```python
from build123d import *

# Parameters (mm, degrees)
PAD002_DEPTH           = 4
SKETCH020_W            = 5
SKETCH020_H            = 30
POCKET003_DEPTH        = 4.001
POCKET003_DEPTH_BACK   = 4.001
FUSION_PLACEMENT_ANGLE = 35


with BuildPart() as obj1:
    # AdditivePipe003: sweep along a path in Sketch015
    with BuildLine(Plane.XZ) as additivepipe003_path:
        Line((0, -9), (10, -9))
        ThreePointArc((10, -9), (19, 2e-06), (9.999996, 9))
        Line((9.999996, 9), (0, 9))
    # Sketch016 → AdditivePipe003 (sweep)
    with BuildSketch(Plane.YZ):
        with BuildLine():
            ThreePointArc((-4, 9), (0, 5), (4, 9))
            Line((4, 11.082268), (4, 9))
            Line((1.261195, 13), (4, 11.082268))
            Line((-1.261195, 13), (1.261195, 13))
            Line((-1.261195, 13), (-4, 11.082268))
            Line((-4, 9), (-4, 11.082268))
        make_face()
    sweep(path=additivepipe003_path.line)

    # AdditivePipe004: sweep along a path in Sketch017
    with BuildLine(Plane.XZ) as additivepipe004_path:
        ThreePointArc((9, 9), (0, 0), (9, -9))
    # Sketch018 → AdditivePipe004 (sweep)
    with BuildSketch(Plane.YZ.offset(9)):
        with BuildLine():
            ThreePointArc((-4, 9), (0, 5), (4, 9))
            Line((4, 11.082268), (4, 9))
            Line((1.261195, 13), (4, 11.082268))
            Line((-1.261195, 13), (1.261195, 13))
            Line((-1.261195, 13), (-4, 11.082268))
            Line((-4, 9), (-4, 11.082268))
        make_face()
    sweep(path=additivepipe004_path.line)

    # Sketch019 → Pad002 (new body, symmetric)
    with BuildSketch(Plane.XZ):
        with BuildLine():
            Line((0, 10), (3.5, 10))
            Line((3.5, 10), (3.5, 8.351647))
            ThreePointArc((3.5, 8.351647), (-1, 0), (3.5, -8.351647))
            Line((3.5, -8.351647), (3.5, -10))
            Line((3.5, -10), (0, -10))
            Line((0, -10), (-2, 0))
            Line((0, 10), (-2, 0))
        make_face()
    extrude(amount=PAD002_DEPTH, both=True)

    # Sketch020 → Pocket003 (cut, two sides)
    with BuildSketch(Plane.XZ) as pocket003_sk:
        with Locations((-2.5, 0)):
            Rectangle(SKETCH020_W, SKETCH020_H)
    extrude(amount=-POCKET003_DEPTH, mode=Mode.SUBTRACT)
    extrude(pocket003_sk.sketch, amount=POCKET003_DEPTH_BACK, mode=Mode.SUBTRACT)


with BuildPart() as fat_link:
    # Part__Mirroring: instance of obj1
    add(obj1.part.mirror(Plane(origin=(0, 0, 0), x_dir=(0, -1, 0), z_dir=(1, 0, 0))))

    # Fusion: union obj1
    add(obj1.part)


with BuildPart() as fat_link_1:
    # Fusion placement: moved
    add(fat_link.part.rotate(Axis((0, 0, 0), (-1, 0, 0)), FUSION_PLACEMENT_ANGLE))


solid = fat_link_1.part
```
Verification items for the finished model (mm, model axes). A direction names the side the tool comes from. Give positions to 0.01 mm unless a question says otherwise; leave off trailing zeros. Use a Markdown table: item, result.
1) Mould release check, pull along X, two halves, no side actions. Record for faces 3 (the cylindrical face through (9.493, 2.94, 4.046)), 4 (the cylindrical face through (-23, 0, 0)), 5 (the flat face through (-0.14, 9.07, 8.33)): pulls with the +X half, pulls with the -X half, needs draft (parallel to the pull), parting line crosses it, or undercut.
Results:
| item | result |
|---|---|
| face 3 | undercut |
| face 4 | pulls with the -X half |
| face 5 | needs draft |
2) Tool access check on faces 1 (the conical face through (-21.17, -3.31, 2.02)), 2 (the cylindrical face through (-9.493, 2.94, 4.046)). Record the directions out of +Z, -Z, +X, -X, +Y, -Y that give a thin tool (end or side, any length) a straight path to the whole face; none if there is none.
Results:
| item | result |
|---|---|
| face 1 | -X, -Y |
| face 2 | none |
3) Material ranges on probe 1 along X at (y, z) = (1, -1.75); probe 2 along X at (y, z) = (-1.5, -1.75); probe 3 along Y at (x, z) = (4.5, 3.25), recorded low to high.
Results:
| item | result |
|---|---|
| probe 1 | -22.58 to -15.37, -3.63 to 3.63, 15.37 to 22.58 |
| probe 2 | -22.8 to -14.45, -4.55 to 4.55, 14.45 to 22.8 |
| probe 3 | 0.34 to 7.02 |
4) Section check A-A, the plane z = -0.5. Give the number of separate pieces and of enclosed holes in the cut face, then the cut area to 3 significant figures.
Results:
| item | result |
|---|---|
| separate pieces | 3 |
| enclosed holes | 0 |
| area | 195 mm² |
5) Depth check by flat-ended pin: pin 1 Ø3 at (y, z) = (-7.5, -2.5) entering from +X; pin 2 Ø6 at (x, z) = (16.5, 5.5) entering from -Y; pin 3 Ø2 at (y, z) = (-4.5, -3) entering from -X. Enter the tip coordinate at first touch or a pass-through.
Results:
| item | result |
|---|---|
| pin 1 | x = 20.04 |
| pin 2 | y = -2.71 |
| pin 3 | x = -22.26 |
